Build history of the part. All positions in model axes, mm. A direction names the side the tool comes from. Round coordinates to 2 decimals unless told otherwise and drop trailing zeros. Write each loop counter-clockwise with the first axis right and the second up, starting at its lowest first coordinate (ties: lowest second). Pieces come first, ordered by that corner, then holes. Notation, with made-up numbers: M 18.5,-6 L 23.5,-6 A18 ccw 23.5,19 Z; hole C 11,57 d3. An arc over 180 degrees is marked long. Write item = value, one per line. Start each with the question number.
Q1. Drop flat-ended pins along their axis: P1, Ø2, axis at x = -2, y = 5.5, coming from the +Z side; P2, Ø2.5, axis at x = 0, z = 0, coming from the +Y side. Give the stop position or say it passes through.
Q2. Band-saw the part on C-C on y = 1.5. Write the cut outline in (x, z) (3 decimals), plus the area to 3 significant figures.
Q3. Band-saw the part on B-B on z = 0. Write the cut outline in (x, y) (3 decimals).
Q4. Pull direction Z, two halves, no side cores. Call faces 1 (the cylindrical face through (0.33, 3.944, -7.493)), 2 (the flat face through (-1, 2, 1)), 3 (the flat face through (-3, 8, 3)): released by +Z, released by -Z, zero draft, split by the parting line, or undercut.
Q5. Band-saw the part on D-D on z = 3. Write the cut outline in (x, y), plus the area to 3 significant figures.
Q6. Tool access for faces 4 (the flat face through (0, 0, 2)), 5 (the cylindrical face through (-3.905, 5.042, -0.867)): list every direction of +Z, -Z, +X, -X, +Y, -Y with a clear straight run to the whole face (end or side of a thin tool).
Q7. Probe L1, parallel to Y at x = -1.75, z = 1; L2, parallel to X at y = 5.5, z = -3; L3, parallel to Z at x = -1, y = 7.5. List the from-to ranges inside material, lowest first.
Q8. Band-saw the part on A-A on x = 0. Write the cut outline in (y, z) (3 decimals).
```python
from build123d import *

# Parameters (mm, degrees)
SKETCH1_R           = 7.5
BOSS_EXTRUDE1_DEPTH = 8
SKETCH2_R           = 4
CUT_EXTRUDE1_DEPTH  = 6
SKETCH3_R           = 1.075
CUT_EXTRUDE2_DEPTH  = 6


with BuildPart() as part:
    # Sketch1 → Boss-Extrude1 (new body)
    with BuildSketch(Plane(origin=(0, 0, 0), x_dir=(1, 0, 0), z_dir=(0, 1, 0))):
        with Locations(Location((0, 0, 0), (0, 0, 270))):  # turned: the seam where the file's is
            Circle(SKETCH1_R)
    extrude(amount=BOSS_EXTRUDE1_DEPTH)

    # Sketch2 → Cut-Extrude1 (cut)
    with BuildSketch(Plane(origin=(0, 8, 0), x_dir=(1, 0, 0), z_dir=(0, 1, 0))):
        with Locations(Location((0, 0, 0), (0, 0, 270))):  # turned: the seam where the file's is
            Circle(SKETCH2_R)
    extrude(amount=-CUT_EXTRUDE1_DEPTH, mode=Mode.SUBTRACT)

    # Sketch3 → Cut-Extrude2 (cut)
    with BuildSketch(Plane.XZ):
        with Locations(Location((0, 0, 0), (0, 0, 270))):  # turned: the seam where the file's is
            Circle(SKETCH3_R)
    extrude(amount=-CUT_EXTRUDE2_DEPTH, mode=Mode.SUBTRACT)


solid = part.part
```
Conclusion:
q1.P1 = 7.43
q1.P2 = 2
q2.outline = C 0,0 d15; hole C 0,0 d2.15
q2.area = 173 mm^2
q3.outline = M -7.5,0 L -1.075,0 L -1.075,2 L -4,2 L -4,8 L -7.5,8 Z; M 1.075,0 L 7.5,0 L 7.5,8 L 4,8 L 4,2 L 1.075,2 Z
q4.face_1 = split by the parting line
q4.face_2 = undercut
q4.face_3 = zero draft
q5.outline = M -6.87,0 L 6.87,0 L 6.87,8 L 2.65,8 L 2.65,2 L -2.65,2 L -2.65,8 L -6.87,8 Z
q5.area = 78.2 mm^2
q6.face_4 = +Z, -Z, +X, -X, -Y
q6.face_5 = +Y
q7.L1 = 0 to 2
q7.L2 = -6.87 to -2.65, 2.65 to 6.87
q7.L3 = -7.43 to -3.87, 3.87 to 7.43
q8.outline = M 0,-7.5 L 8,-7.5 L 8,-4 L 2,-4 L 2,-1.075 L 0,-1.075 Z; M 0,1.075 L 2,1.075 L 2,4 L 8,4 L 8,7.5 L 0,7.5 Z
